Part print with two shaded views. Sizes in mm from the minimum x, y, z corner. A direction names the side the tool comes from. Round coordinates to 2 decimals unless told otherwise and drop trailing zeros. Write each loop counter-clockwise with the first axis right and the second up, starting at its lowest first coordinate (ties: lowest second). Pieces come first, ordered by that corner, then holes. Notation, with made-up numbers: (0.5, 44.25) - (45.5, 44.25) arc R17 ccw to (45.5, 62.25) - close; hole circle Ø11 at (32.5, 47.25). An arc over 180 degrees is marked (long way). Use one line per item in the form item = value. Start each with the question number.
Item 1: Band-saw the part on C-C, the plane z = 23. List the corners of the cut face in (x, y), and give its area (3 significant figures).
Item 2: Pin check, flat tips, straight feed: pin 1 (12 mm diameter, centred on y = 9, z = 36, fed in from +X); pin 2 (11.5 mm diameter, centred on x = 25.4, y = 12.7, fed in from -Z) (1 decimal). Stop position of each tip, or through.
Item 3: Band-saw the part on A-A, the plane x = 25.4. List the corners of the cut face in (y, z).
Item 4: Pull direction X, two halves, no side cores. Call the marked faces 4, 5, 6 and 7: +X half, -X half, draft (parallel to the pull), parting line (faces both ways), or undercut.
Item 5: Band-saw the part on B-B, the plane y = 16. List the corners of the cut face in (x, z) (1 decimal).
Item 6: Drill centre lines: L1, parallel to Y at x = 25, z = 3; L2, parallel to Y at x = 5, z = 33; L3, parallel to Z at x = 35, y = 10.75. Where is each one in solid material? Low to high.
Item 7: Band-saw the part on D-D, the plane x = 48. List the corners of the cut face in (y, z) (1 decimal), and give its area (3 significant figures).
Item 8: Tool access for the marked faces 1, 2 and 3: list every direction of +Z, -Z, +X, -X, +Y, -Y with a clear straight run to the whole face (end or side of a thin tool).
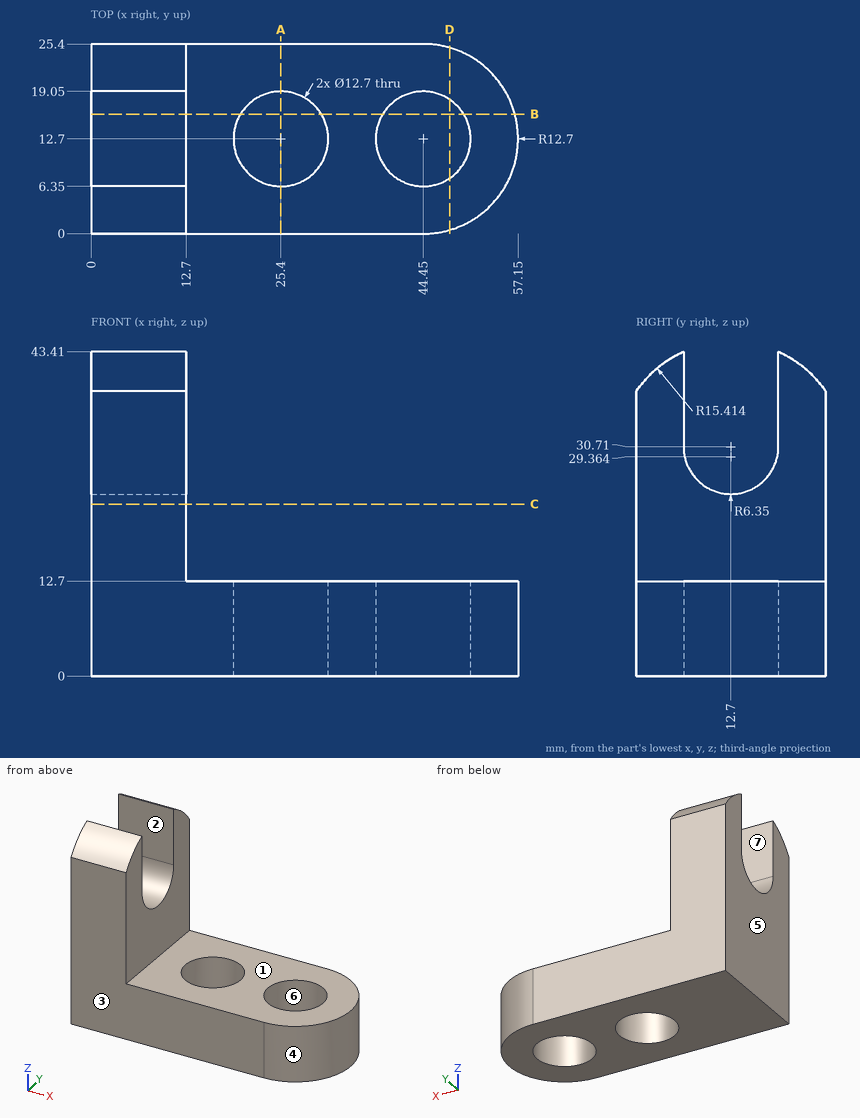
Determined:
q1.outline = (0, 0) - (12.7, 0) - (12.7, 25.4) - (0, 25.4) - close
q1.area = 323 mm²
q2.pin_1 = 12.7
q2.pin_2 = through
q3.outline = (0, 0) - (6.35, 0) - (6.35, 12.7) - (0, 12.7) - close; (19.05, 0) - (25.4, 0) - (25.4, 12.7) - (19.05, 12.7) - close
q4.face_4 = +X half
q4.face_5 = -X half
q4.face_6 = undercut
q4.face_7 = draft
q5.outline = (0, 0) - (20, 0) - (20, 12.7) - (12.7, 12.7) - (12.7, 25.3) - (0, 25.3) - close; (30.8, 0) - (39, 0) - (39, 12.7) - (30.8, 12.7) - close; (49.9, 0) - (56.7, 0) - (56.7, 12.7) - (49.9, 12.7) - close
q6.L1 = 0 to 6.36, 19.04 to 25.4
q6.L2 = 0 to 6.35, 19.05 to 25.4
q6.L3 = 0 to 12.7
q7.outline = (0.5, 0) - (7.4, 0) - (7.4, 12.7) - (0.5, 12.7) - close; (18, 0) - (24.9, 0) - (24.9, 12.7) - (18, 12.7) - close
q7.area = 176 mm²
q8.face_1 = +Z, +X, +Y, -Y
q8.face_2 = +Z, +X, -X
q8.face_3 = +Z, -Z, +X, -X, -Y
